Part model, mm, in its own coordinate system. Face numbers are marked on the shaded views. A direction names the side the tool comes from. Coordinates: 2 decimals unless noted, no trailing zeros. Write each loop counter-clockwise with the first axis right and the second up, starting at its lowest first coordinate (ties: lowest second). Pieces come first, ordered by that corner, then holes. Notation, with made-up numbers: (87.25, 7.25) - (98.25, 7.25) arc R13 cw to (98.25, 20.25) - close; hole circle Ø6 at (52.25, 86). An arc over 180 degrees is marked (long way). Use one line per item in the form item = value. Start each with the question number.
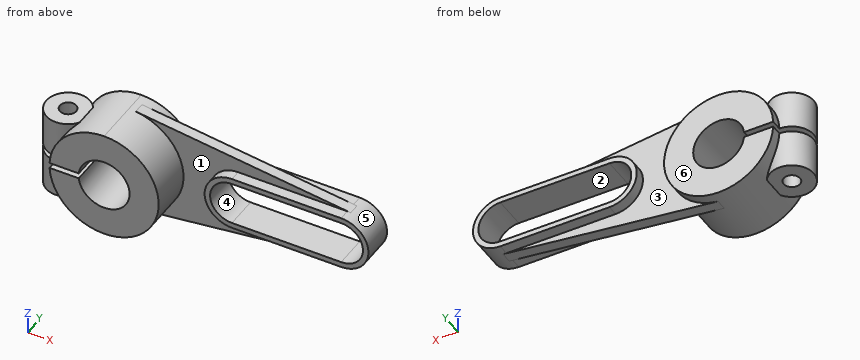
from build123d import *

# Parameters (mm, degrees)
SKETCH1_R           = 30
SKETCH1_R_2         = 14
BOSS_EXTRUDE1_DEPTH = 36
BOSS_EXTRUDE2_DEPTH = 18
BOSS_EXTRUDE3_START = -12
BOSS_EXTRUDE3_DEPTH = 6
CUT_EXTRUDE1_DEPTH  = 143.902064366
SKETCH5_R           = 12
BOSS_EXTRUDE4_DEPTH = 22.4
CUT_EXTRUDE2_DEPTH  = 143.902064412
HOLE1_D             = 9


with BuildPart() as part:
    # Sketch1 → Boss-Extrude1 (new body)
    with BuildSketch(Plane(origin=(0, 0, 0), x_dir=(1, 0, 0), z_dir=(0, 1, 0))):
        with Locations(Location((0, 0, 0), (0, 0, 270))):
            Circle(SKETCH1_R)
        with Locations(Location((0, 0, 0), (0, 0, 270))):
            Circle(SKETCH1_R_2, mode=Mode.SUBTRACT)
    extrude(amount=BOSS_EXTRUDE1_DEPTH)



with BuildPart() as body_2:
    # Sketch2 → Boss-Extrude2 (new body)
    with BuildSketch(Plane(origin=(0, 36, 0), x_dir=(1, 0, 0), z_dir=(0, 1, 0))):
        with BuildLine():
            Line((60, 15), (120, 15))
            ThreePointArc((120, 15), (135, 0), (120, -15))
            Line((120, -15), (60, -15))
            ThreePointArc((60, -15), (45, 0), (60, 15))
        make_face()
    extrude(amount=-BOSS_EXTRUDE2_DEPTH)


with BuildPart() as part_1:
    add(part.part)

    add(body_2.part)  # Boss-Extrude3 merges body 2
    # Sketch3 → Boss-Extrude3 (add)
    with BuildSketch(Plane(origin=(0, 36, 0), x_dir=(1, 0, 0), z_dir=(0, 1, 0)).offset(BOSS_EXTRUDE3_START)):
        with BuildLine():
            Line((3.75, -29.764702249), (121.875, -14.882351125))
            ThreePointArc((121.875, -14.882351125), (135, 0), (121.875, 14.882351125))
            Line((121.875, 14.882351125), (3.75, 29.764702249))
            ThreePointArc((3.75, 29.764702249), (30, 0), (3.75, -29.764702249))
        make_face()
    extrude(amount=BOSS_EXTRUDE3_DEPTH)

    # Sketch4 → Cut-Extrude1 (cut, through all)
    with BuildSketch(Plane(origin=(0, 36, 0), x_dir=(1, 0, 0), z_dir=(0, 1, 0))):
        with BuildLine():
            Line((60, 12), (120, 12))
            ThreePointArc((120, 12), (132, 0), (120, -12))
            Line((120, -12), (60, -12))
            ThreePointArc((60, -12), (48, 0), (60, 12))
        make_face()
    extrude(amount=-CUT_EXTRUDE1_DEPTH, mode=Mode.SUBTRACT)

    # Sketch5 → Boss-Extrude4 (add, symmetric)
    with BuildSketch(Plane.XY):
        with Locations((-30, 18)):
            Circle(SKETCH5_R)
    extrude(amount=BOSS_EXTRUDE4_DEPTH, both=True)

    # Sketch6 → Cut-Extrude2 (cut, through all)
    with BuildSketch(Plane(origin=(0, 36, 0), x_dir=(1, 0, 0), z_dir=(0, 1, 0))):
        with BuildLine():
            Line((-45, 1.5), (-13.919410907, 1.5))
            ThreePointArc((-13.919410907, 1.5), (-14, 0), (-13.919410907, -1.5))
            Line((-13.919410907, -1.5), (-45, -1.5))
            Line((-45, -1.5), (-45, 1.5))
        make_face()
    extrude(amount=-CUT_EXTRUDE2_DEPTH, mode=Mode.SUBTRACT)

    # Hole1 (through all)
    with Locations(Plane.XY.offset(22.4)):
        with Locations((-30, 18)):
            Hole(HOLE1_D / 2)


solid = part_1.part
Q1. Mould opens along Z. For the marked faces 4, 5 and 6 say: released by +Z, released by -Z, zero draft, split by the parting line, or undercut.
Q2. Slice it at A-A (z = -10). List the corners of the cut face in (x, y).
Q3. Drill centre lines: probe 1 along Y at (x, z) = (-30, 12.5); probe 2 along Z at (x, y) = (-30, 27.5); probe 3 along X at (y, z) = (23, -7). Where is each one in solid material? Low to high.
Q4. Pin check, flat tips, straight feed: P1, Ø12, axis at y = 25.5, z = 11.5, coming from the +X side; P2, Ø8, axis at x = 45, y = 29.5, coming from the +Z side; P3, Ø12, axis at x = 50, z = -15, coming from the -Y side. Stop position of each tip, or through.
Q5. Slice it at C-C (z = -20). List the corners of the cut face in (x, y).
Q6. Slice it at B-B (x = 73). List the corners of the cut face in (y, z).
Q7. Which spindle directions (+Z, -Z, +X, -X, +Y, -Y) get a long thin tool onto all of the face, cutting with end or side? Do the marked faces 1, 2 and 3. Say none if no direction does.
Q8. Slice it at D-D (y = 3.5). List the corners of the cut face in (x, z).
Solution:
q1.face_4 = undercut
q1.face_5 = split by the parting line
q1.face_6 = zero draft
q2.outline = (-28.28, 0) - (-9.8, 0) - (-9.8, 36) - (-28.28, 36) - (-28.28, 29.88) arc R12 ccw (long way) to (-28.28, 6.12) - close; (9.8, 0) - (28.28, 0) - (28.28, 24) - (48.82, 24) - (48.82, 18) - (53.37, 18) - (53.37, 36) - (48.82, 36) - (48.82, 30) - (28.28, 30) - (28.28, 36) - (9.8, 36) - close; (126.63, 18) - (131.18, 18) - (131.18, 36) - (126.63, 36) - close; hole circle Ø9 at (-30, 18)
q3.probe_1 = 6 to 13.5, 22.5 to 30
q3.probe_2 = -22.4 to -1.5, 1.5 to 22.4
q3.probe_3 = -40.91 to -12.12, 12.12 to 29.17, 46.73 to 50.25, 129.75 to 133.27
q4.P1 = 133.96
q4.P2 = 25.07
q4.P3 = 18
q5.outline = (-22.36, 0) - (22.36, 0) - (22.36, 24) - (81.25, 24) - (81.25, 30) - (22.36, 30) - (22.36, 36) - (-22.36, 36) - (-22.36, 27.25) arc R12 ccw (long way) to (-22.36, 8.75) - close; hole circle Ø9 at (-30, 18)
q6.outline = (18, -15) - (24, -15) - (24, -21.04) - (30, -21.04) - (30, -15) - (36, -15) - (36, -12) - (18, -12) - close; (18, 12) - (36, 12) - (36, 15) - (30, 15) - (30, 21.04) - (24, 21.04) - (24, 15) - (18, 15) - close
q7.face_1 = -Y
q7.face_2 = +Y, -Y
q7.face_3 = +Y
q8.outline = (-29.96, -1.5) arc R30 ccw (long way) to (-29.96, 1.5) - (-13.92, 1.5) arc R14 cw (long way) to (-13.92, -1.5) - close
